Geometry check sheet. Reference: drawing and pictorial views, mm from the part's lowest x, y, z. Coordinates: 2 decimals unless noted, no trailing zeros. Write each loop counter-clockwise with the first axis right and the second up, starting at its lowest first coordinate (ties: lowest second). Pieces come first, ordered by that corner, then holes. Notation, with made-up numbers: (26.5, 44.25) -> (38.5, 44.25) arc R31 cw to (38.5, 71.25) -> close; hole circle Ø7 at (-35, -17.5). An arc over 180 degrees is marked (long way). Answer in a Markdown table with one row per item.
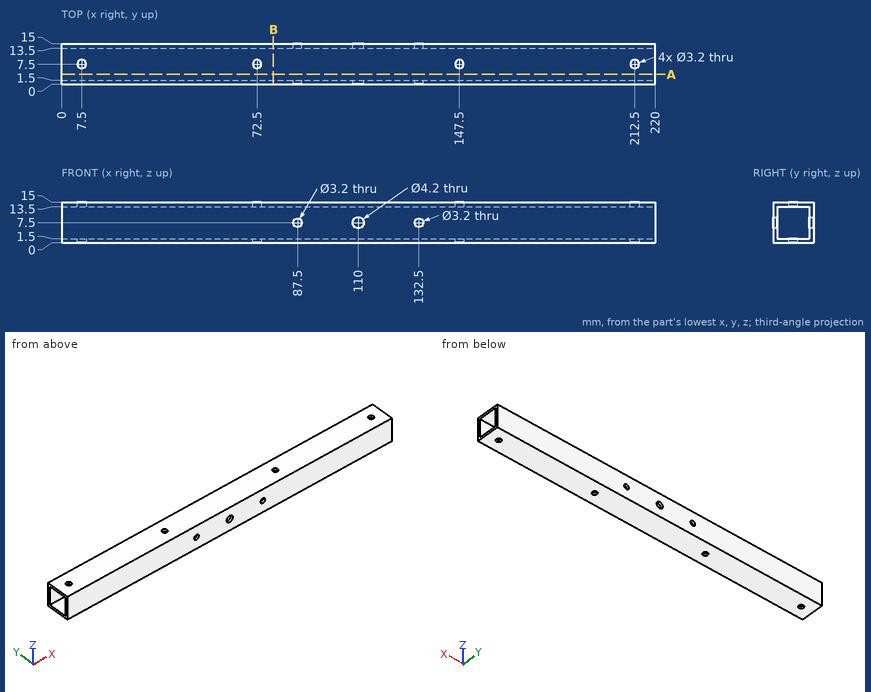
1. Section check B-B, the plane x = 78.5. Record the boundary of the cut face in (y, z), plus the area to 3 significant figures.
Geometry says:
| item | result |
|---|---|
| outline | (0, 0) -> (15, 0) -> (15, 15) -> (0, 15) -> close; hole (1.5, 1.5) -> (13.5, 1.5) -> (13.5, 13.5) -> (1.5, 13.5) -> close |
| area | 81.0 mm^2 |
2. Section check A-A, the plane y = 3.75. Record the boundary of the cut face in (x, z).
Geometry says:
| item | result |
|---|---|
| outline | (0, 0) -> (220, 0) -> (220, 1.5) -> (0, 1.5) -> close; (0, 13.5) -> (220, 13.5) -> (220, 15) -> (0, 15) -> close |
3. Depth check by flat-ended pin: P1, Ø3.5, axis at x = 110, z = 7.5, coming from the +Y side (3 decimals). Enter the tip coordinate at first touch or a pass-through.
Geometry says:
| item | result |
|---|---|
| P1 | through |
4. Thickness scan on line 1 (X direction, y = 14.15, z = 7.5); line 2 (Y direction, x = 177, z = 3.5). Record the ranges inside material, lowest first. Write a range as from..to.
Geometry says:
| item | result |
|---|---|
| line 1 | 0..85.9, 89.1..107.9, 112.1..130.9, 134.1..220 |
| line 2 | 0..1.5, 13.5..15 |
